Design review of the part built by this model. Coordinates are the model's own, in mm. Give positions to 0.01 mm unless a question says otherwise; leave off trailing zeros. Order: outer loops, then holes, each group sorted by start corner. A loop starts at its lowest first (then second) coordinate and runs counter-clockwise, first axis right, second up. Notation, with made-up numbers: (53, 63) -> (86, 63) arc R32 ccw to (86, 93) -> close; hole circle Ø9 at (16.5, -13). An arc over 180 degrees is marked (long way). Use a Markdown table: item, result. Add a question column.
```python
from build123d import *

# Parameters (mm, degrees)
F0_W     = 254
F0_H     = 127
F1_DEPTH = 50.8
F2_W     = 121.92
F2_H     = 45.72
F3_DEPTH = 254.001
F5_D     = 5.1054


with BuildPart() as f1:
    # F0 (on Top) → F1 (new body)
    with BuildSketch(Plane.XY):
        with Locations((3.112221, 47.606194)):
            Rectangle(F0_W, F0_H)
    extrude(amount=F1_DEPTH)

    # F2 (on face) → F3 (cut, through all)
    with BuildSketch(Plane.YZ.offset(130.112221)):
        with Locations((47.606194, 25.4)):
            Rectangle(F2_W, F2_H)
    extrude(amount=-F3_DEPTH, mode=Mode.SUBTRACT)

    # F5 (through all)
    with Locations(Plane.XY.offset(50.8)):
        with Locations((-60.387779, 47.606194), (15.812221, 73.006194), (41.212221, 98.406194), (-111.187779, 47.606194), (-34.987779, 73.006194), (-60.387779, 22.206194), (15.812221, 47.606194), (41.212221, 73.006194), (-85.787779, 73.006194), (-111.187779, 22.206194), (-9.587779, 98.406194), (-34.987779, 47.606194), (-60.387779, 98.406194), (41.212221, -3.193806), (66.612221, 47.606194), (-85.787779, -3.193806), (-9.587779, 22.206194), (-60.387779, -3.193806), (15.812221, 22.206194), (92.012221, -3.193806), (41.212221, 47.606194), (66.612221, 98.406194), (-111.187779, -3.193806), (-85.787779, 47.606194), (-34.987779, 22.206194), (-9.587779, 73.006194), (66.612221, 73.006194), (66.612221, 22.206194), (117.412221, 98.406194), (117.412221, 73.006194), (117.412221, 47.606194), (117.412221, 22.206194), (117.412221, -3.193806), (92.012221, 98.406194), (92.012221, 73.006194), (92.012221, 47.606194), (92.012221, 22.206194), (-111.187779, 98.406194), (-9.587779, -3.193806), (-85.787779, 98.406194), (15.812221, -3.193806), (-60.387779, 73.006194), (15.812221, 98.406194), (41.212221, 22.206194), (-85.787779, 22.206194), (-9.587779, 47.606194), (-34.987779, -3.193806), (66.612221, -3.193806), (-111.187779, 73.006194), (-34.987779, 98.406194)):
            Hole(F5_D / 2)


solid = f1.part
```
1) Add section C-C (z = 16). Give the boundary of the cut face in (x, y).
2) The part is to be moulded in two halves that separate along X. For faces 1 (the flat face through (5, 108.566, 25)), 2 (the cylindrical face through (66.945, 24.737, 49.512)), say which applies: +X half, -X half, draft (parallel to the pull), parting line (faces both ways), or undercut.
3) Insertion check: pin 1 (3 mm diameter, centred on x = -85.79, y = 47.61, fed in from +Z); pin 2 (2 mm diameter, centred on x = 62.5, y = 2, fed in from -Z). Each pin has a flat end and moves straight along its axis. Give the tip position at first contact, or say it passes through.
4) Add section A-A (y = 89). Give the boundary of the cut face in (x, z).
5) For L1, parallel to Y at x = -29.5, z = 16.5; L2, parallel to Z at x = -76, y = 11.5, list the stretches that pass through material, from the lowest coordinate up. Write a range as [from, to].
6) Add section B-B (x = -41). Give the boundary of the cut face in (y, z).
Worked answers:
| question | item | result |
|---|---|---|
| 1 | outline | (-123.89, -15.89) -> (130.11, -15.89) -> (130.11, -13.35) -> (-123.89, -13.35) -> close; (-123.89, 108.57) -> (130.11, 108.57) -> (130.11, 111.11) -> (-123.89, 111.11) -> close |
| 2 | face 1 | draft |
| 2 | face 2 | undercut |
| 3 | pin 1 | through |
| 3 | pin 2 | z = 0 |
| 4 | outline | (-123.89, 0) -> (130.11, 0) -> (130.11, 2.54) -> (-123.89, 2.54) -> close; (-123.89, 48.26) -> (130.11, 48.26) -> (130.11, 50.8) -> (-123.89, 50.8) -> close |
| 5 | L1 | [-15.89, -13.35], [108.57, 111.11] |
| 5 | L2 | [0, 2.54], [48.26, 50.8] |
| 6 | outline | (-15.89, 0) -> (111.11, 0) -> (111.11, 50.8) -> (-15.89, 50.8) -> close; hole (-13.35, 2.54) -> (108.57, 2.54) -> (108.57, 48.26) -> (-13.35, 48.26) -> close |
